Design review of the part built by this model. Coordinates are the model's own, in mm. Face numbers are marked on the shaded views. Round coordinates to 2 decimals unless told otherwise and drop trailing zeros. Write each loop counter-clockwise with the first axis right and the second up, starting at its lowest first coordinate (ties: lowest second). Pieces come first, ordered by that corner, then holes. Notation, with made-up numbers: M 43.5,-33.5 L 58.5,-33.5 A13 ccw 58.5,-12.5 Z; hole C -20.5,19.5 d5. An arc over 180 degrees is marked long. Use CSV: the item, a comma, the result in double quotes.
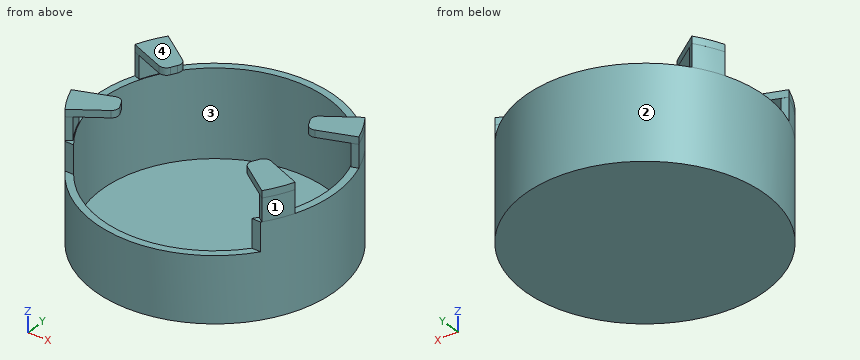
from build123d import *

# Parameters (mm, degrees)
SKETCH007_R                    = 8.5
PAD006_DEPTH                   = 6.6
THICKNESS_T                    = -0.5
PAD007_DEPTH                   = 1.6
PAD007_POLARPATTERN_2_DEPTH    = 1.6
PAD008_DEPTH                   = 0.5
PAD008_POLARPATTERN001_2_DEPTH = 0.5
SKETCH011_W                    = 13.925584
SKETCH011_H                    = 6.6246
POCKET001_DEPTH                = 2
FILLET006_R                    = 0.5


with BuildPart() as part:
    # Sketch007 (on DatumPlane) → Pad006 (new body)
    with BuildSketch(Plane(origin=(0, 0, -1), x_dir=(1, 0, 0), z_dir=(0, 0, -1))):
        Circle(SKETCH007_R)
    extrude(amount=PAD006_DEPTH)

    # Thickness
    thickness_openings = [part.faces().sort_by_distance(p)[0] for p in [
        (0, 0, -1),
    ]]
    offset(amount=THICKNESS_T, openings=thickness_openings)

    # Sketch008 (on Face3 of Thickness) → Pad007 (join)
    with BuildSketch(Plane.XY.offset(-1)):
        with BuildLine():
            ThreePointArc((-7.005526, 4.813794), (-7.541696, 3.920819), (-7.964623, 2.96897))
            Line((-7.540357, 2.810816), (-7.964623, 2.96897))
            ThreePointArc((-6.632349, 4.557368), (-7.139959, 3.711961), (-7.540357, 2.810816))
            Line((-6.632349, 4.557368), (-7.005526, 4.813794))
        make_face()
    pad007 = extrude(amount=PAD007_DEPTH)

    # Sketch008 PolarPattern 2 → Pad007 PolarPattern 2 (add)
    with BuildSketch(Plane(origin=(0, 0, -1), x_dir=(-1, 0, 0), z_dir=(0, 0, 1))):
        with BuildLine():
            ThreePointArc((-7.005526, 4.813794), (-7.541696, 3.920819), (-7.964623, 2.96897))
            Line((-7.540357, 2.810816), (-7.964623, 2.96897))
            ThreePointArc((-6.632349, 4.557368), (-7.139959, 3.711961), (-7.540357, 2.810816))
            Line((-6.632349, 4.557368), (-7.005526, 4.813794))
        make_face()
    pad007_polarpattern_2 = extrude(amount=PAD007_POLARPATTERN_2_DEPTH)

    # Mirrored: Pad007, Pad007 PolarPattern 2 across Sketch008 V_Axis
    add(pad007.mirror(Plane(origin=(0, 0, -1), x_dir=(0, 0, 1), z_dir=(1, 0, 0))))
    add(pad007_polarpattern_2.mirror(Plane(origin=(0, 0, -1), x_dir=(0, 0, 1), z_dir=(1, 0, 0))))

    # Sketch009 (on Face23 of MultiTransform) → Pad008 (join)
    with BuildSketch(Plane.XY.offset(0.6)):
        with BuildLine():
            ThreePointArc((-7.005526, 4.813794), (-7.542066, 3.921011), (-7.964623, 2.96897))
            Line((-5.09111, 1.862853), (-7.964623, 2.96897))
            ThreePointArc((-4.469489, 3.068188), (-4.818529, 2.485236), (-5.09111, 1.862853))
            Line((-7.005526, 4.813794), (-4.469489, 3.068188))
        make_face()
    pad008 = extrude(amount=PAD008_DEPTH)

    # Sketch009 PolarPattern001 2 → Pad008 PolarPattern001 2 (add)
    with BuildSketch(Plane(origin=(0, 0, 0.6), x_dir=(-1, 0, 0), z_dir=(0, 0, 1))):
        with BuildLine():
            ThreePointArc((-7.005526, 4.813794), (-7.542066, 3.921011), (-7.964623, 2.96897))
            Line((-5.09111, 1.862853), (-7.964623, 2.96897))
            ThreePointArc((-4.469489, 3.068188), (-4.818529, 2.485236), (-5.09111, 1.862853))
            Line((-7.005526, 4.813794), (-4.469489, 3.068188))
        make_face()
    pad008_polarpattern001_2 = extrude(amount=PAD008_POLARPATTERN001_2_DEPTH)

    # Mirrored001: Pad008, Pad008 PolarPattern001 2 across Sketch009 V_Axis
    add(pad008.mirror(Plane(origin=(0, 0, 0.6), x_dir=(0, 0, 1), z_dir=(1, 0, 0))))
    add(pad008_polarpattern001_2.mirror(Plane(origin=(0, 0, 0.6), x_dir=(0, 0, 1), z_dir=(1, 0, 0))))

    # Sketch011 (on Face1 of ShapeBinder001) → Pocket001 (cut)
    with BuildSketch(Plane(origin=(0, 0, -1), x_dir=(1, 0, 0), z_dir=(0, 0, -1))):
        with Locations((0, 8.1877)):
            Rectangle(SKETCH011_W, SKETCH011_H)
    extrude(amount=POCKET001_DEPTH, mode=Mode.SUBTRACT)

    # Fillet006
    fillet006_edges = [part.edges().sort_by_distance(p)[0] for p in [
        (-5.09111, -1.862853, 0.85),
        (-4.469489, -3.068188, 0.85),
        (4.469489, -3.068188, 0.85),
        (5.09111, -1.862853, 0.85),
        (5.09111, 1.862853, 0.85),
        (4.469489, 3.068188, 0.85),
        (-5.09111, 1.862853, 0.85),
        (-4.469489, 3.068188, 0.85),
    ]]
    fillet(fillet006_edges, radius=FILLET006_R)


solid = part.part
1) The part is to be moulded in two halves that separate along X. For the marked faces 1, 2, 3 and 4, say which applies: released by +X, released by -X, zero draft, split by the parting line, or undercut.
Answers:
face 1,"released by +X"
face 2,"split by the parting line"
face 3,"undercut"
face 4,"zero draft"
2) Add section C-C on z = -6.5. Write out the cut boundary in (x, y).
Answers:
outline,"C 0,0 d17; hole C 0,0 d16"
3) Add section A-A on x = 0. Write out the cut boundary in (y, z), then the cut area to 3 significant figures.
Answers:
outline,"M -8.5,-7.6 L 8.5,-7.6 L 8.5,-1 L 8,-1 L 8,-7.1 L -8,-7.1 L -8,-3 L -8.5,-3 Z"
area,"13.6 mm²"
4) Add section B-B on y = 0. Write out the cut boundary in (x, z), then the cut area to 3 significant figures.
Answers:
outline,"M -8.5,-7.6 L 8.5,-7.6 L 8.5,-1 L 8,-1 L 8,-7.1 L -8,-7.1 L -8,-1 L -8.5,-1 Z"
area,"14.6 mm²"
5) For pin 1 Ø1 at (x, z) = (-6.5, -3) entering from +Y; pin 2 Ø1.5 at (x, z) = (4, -5.5) entering from -Y; pin 3 Ø0.5 at (x, z) = (6.5, -2) entering from -Y, all flat-tipped, find the tip position at first contact; note any pin that passes through.
Answers:
pin 1,"y = 6.02"
pin 2,"y = -7.85"
pin 3,"y = -4.88"
6) Wall thickness on line 1 along Y through (x, z) = (0, -3.75); line 2 along Z through (x, y) = (5.5, 3.5): over which ranges is each line inside the solid? List them lowest first. Write a range as [from, to].
Answers:
line 1,"[-8.5, -8], [8, 8.5]"
line 2,"[-7.6, -7.1], [0.6, 1.1]"
7) Add section D-D on z = -1.75. Write out the cut boundary in (x, y), then the cut area to 3 significant figures.
Answers:
outline,"M -6.96,-4.88 L -6.34,-4.88 A8 cw long 6.34,-4.88 L 6.96,-4.88 A8.5 ccw long Z"
area,"18.2 mm²"
